Design review of the part built by this model. Coordinates are the model's own, in mm. A direction names the side the tool comes from. Coordinates: 2 decimals unless noted, no trailing zeros. Order: outer loops, then holes, each group sorted by start corner. A loop starts at its lowest first (then second) coordinate and runs counter-clockwise, first axis right, second up. Notation, with made-up numbers: M -31,20 L 3,20 A22 cw 3,48 Z; hole C -12.75,21 d2. An arc over 180 degrees is marked long. Answer as a JSON object with one key per item and string values.
from build123d import *

# Parameters (mm, degrees)
BOSS_EXTRUDE1_DEPTH = 90
FILLET1_R           = 15
CUT_EXTRUDE1_START  = -15
CUT_EXTRUDE1_DEPTH  = 600


with BuildPart() as part:
    # Sketch1 → Boss-Extrude1 (new body)
    with BuildSketch(Plane.XY):
        with BuildLine():
            Line((-120, 0), (120, 0))
            Line((120, 0), (120, -70))
            Line((120, -70), (80, -70))
            ThreePointArc((80, -70), (0, -92.643375225), (-80, -70))
            Line((-80, -70), (-120, -70))
            Line((-120, -70), (-120, 0))
        make_face()
    extrude(amount=-BOSS_EXTRUDE1_DEPTH)

    # Fillet1
    fillet1_edges = [part.edges().sort_by_distance(p)[0] for p in [
        (-120, -70, -45),
        (-80, -70, -45),
        (80, -70, -45),
        (120, -70, -45),
        (100, -70, -90),
        (0, -92.643375225, -90),
        (-100, -70, -90),
        (-100, -70, 0),
        (0, -92.643375225, 0),
        (100, -70, 0),
    ]]
    fillet(fillet1_edges, radius=FILLET1_R)


with BuildPart() as body_2:
    # Body-Move/Copy1: read off the stored shape, not the designer's step
    # Body-Move/Copy1: copy of part
    add(part.part.moved(Location((0, 0, -540))))


with BuildPart() as body_3:
    # Body-Move_Copy1 2: copy of part
    add(part.part.moved(Location((0, 0, -450))))


with BuildPart() as body_4:
    # Body-Move_Copy1 3: copy of part
    add(part.part.moved(Location((0, 0, -360))))


with BuildPart() as body_5:
    # Body-Move_Copy1 4: copy of part
    add(part.part.moved(Location((0, 0, -270))))


with BuildPart() as body_6:
    # Body-Move_Copy1 5: copy of part
    add(part.part.moved(Location((0, 0, -180))))


with BuildPart() as body_7:
    # Body-Move_Copy1 6: copy of part
    add(part.part.moved(Location((0, 0, -90))))


with BuildPart() as part_1:
    add(part.part)

    # Combine1: union body 7, body 6, body 5, body 4, body 3, body 2
    add(body_7.part)
    add(body_6.part)
    add(body_5.part)
    add(body_4.part)
    add(body_3.part)
    add(body_2.part)

    # Sketch2 → Cut-Extrude1 (cut)
    with BuildSketch(Plane(origin=(0, 0, -630), x_dir=(-1, 0, 0), z_dir=(0, 0, -1)).offset(CUT_EXTRUDE1_START)):
        with BuildLine():
            Line((-110, -10), (-110, 0))
            Line((-110, 0), (110, 0))
            Line((110, 0), (110, -10))
            Line((110, -10), (110, -45))
            Line((110, -45), (84.138583639, -45))
            ThreePointArc((84.138583639, -45), (73.743634299, -46.374295758), (64.062971697, -50.402748589))
            ThreePointArc((64.062971697, -50.402748589), (0, -67.643375225), (-64.062971697, -50.402748589))
            ThreePointArc((-64.062971697, -50.402748589), (-73.743634299, -46.374295758), (-84.138583639, -45))
            Line((-84.138583639, -45), (-110, -45))
            Line((-110, -45), (-110, -10))
        make_face()
    extrude(amount=-CUT_EXTRUDE1_DEPTH, mode=Mode.SUBTRACT)


solid = part_1.part
1) Add section B-B (z = -237). State the section outline as (x, y) points, and give its area (3 significant figures).
Taken from the geometry:
{"outline": "M -120,-55 A15 ccw -105,-70 L -84.14,-70 A15 cw -76.61,-72.03 A152.64 ccw 76.61,-72.03 A15 cw 84.14,-70 L 105,-70 A15 ccw 120,-55 L 120,0 L 110,0 L 110,-45 L 84.14,-45 A40 ccw 64.06,-50.4 A127.64 cw -64.06,-50.4 A40 ccw -84.14,-45 L -110,-45 L -110,0 L -120,0 Z", "area": "7,000 mm2"}
2) Mouldability with a two-part tool opening along X and no side actions: class faces 1 (the cylindrical face through (1.12, -92.64, -584.58)), 2 (the cylindrical face through (-115.49, -65.72, -315.63)), 3 (the flat face through (110, -23, -319)) as released by +X, released by -X, zero draft, split by the parting line, or undercut.
Taken from the geometry:
{"face 1": "split by the parting line", "face 2": "released by -X", "face 3": "undercut"}
3) Insertion check: pin 1 Ø10.5 at (x, z) = (-96, -414) entering from -Y; pin 2 Ø13 at (x, z) = (100, -171) entering from +Y; pin 3 Ø2 at (x, z) = (13.5, -437) entering from -Y. Each pin has a flat end and moves straight along its axis. Give the tip position at first contact, or say it passes through.
Taken from the geometry:
{"pin 1": "stops at y = -70", "pin 2": "stops at y = -45", "pin 3": "stops at y = -92.05"}
4) Add section A-A (y = -18.5). State the section outline as (x, z) points, and give its area (3 significant figures).
Taken from the geometry:
{"outline": "M -120,-630 L 120,-630 L 120,0 L -120,0 Z; hole M -110,-615 L 110,-615 L 110,-15 L -110,-15 Z", "area": "19,200 mm2"}
5) To check wall thickness, follow L1, parallel to X at y = -17.5, z = -344; L2, parallel to Z at x = 86, y = -35; L3, parallel to X at y = -58, z = -186. State the ranges of each line that lie inside material, in increasing order.
Taken from the geometry:
{"L1": "x = -120 to -110, 110 to 120", "L2": "z = -630 to -615, -15 to 0", "L3": "x = -119.7 to -48.67, 48.67 to 119.7"}
6) Tool access review of faces 4 (the flat face through (95, -70, -45)), 5 (the flat face through (-94, -70, -495)), 6 (the flat face through (-97, -45, -319)): name each direction out of +Z, -Z, +X, -X, +Y, -Y from which nothing blocks a thin tool from reaching the whole face with its end or side.
Taken from the geometry:
{"face 4": "+Z, -Z, +X, -Y", "face 5": "+Z, -Z, -X, -Y", "face 6": "+Y"}
7) Add section C-C (y = -84.5). Count the separate pieces of the cut face and the enclosed holes in it, and give its area (3 significant figures).
Taken from the geometry:
{"separate pieces": "7", "enclosed holes": "0", "area": "56,400 mm2"}
